Input: dimensioned drawing with shaded views. Units: mm. Origin: part minimum x, y, z. A direction names the side the tool comes from. Give positions to 0.01 mm unless a question says otherwise; leave off trailing zeros. Loops run counter-clockwise (first coordinate to the right, second up) from the corner with the lowest first, then second, coordinate; pieces in that order, holes last.
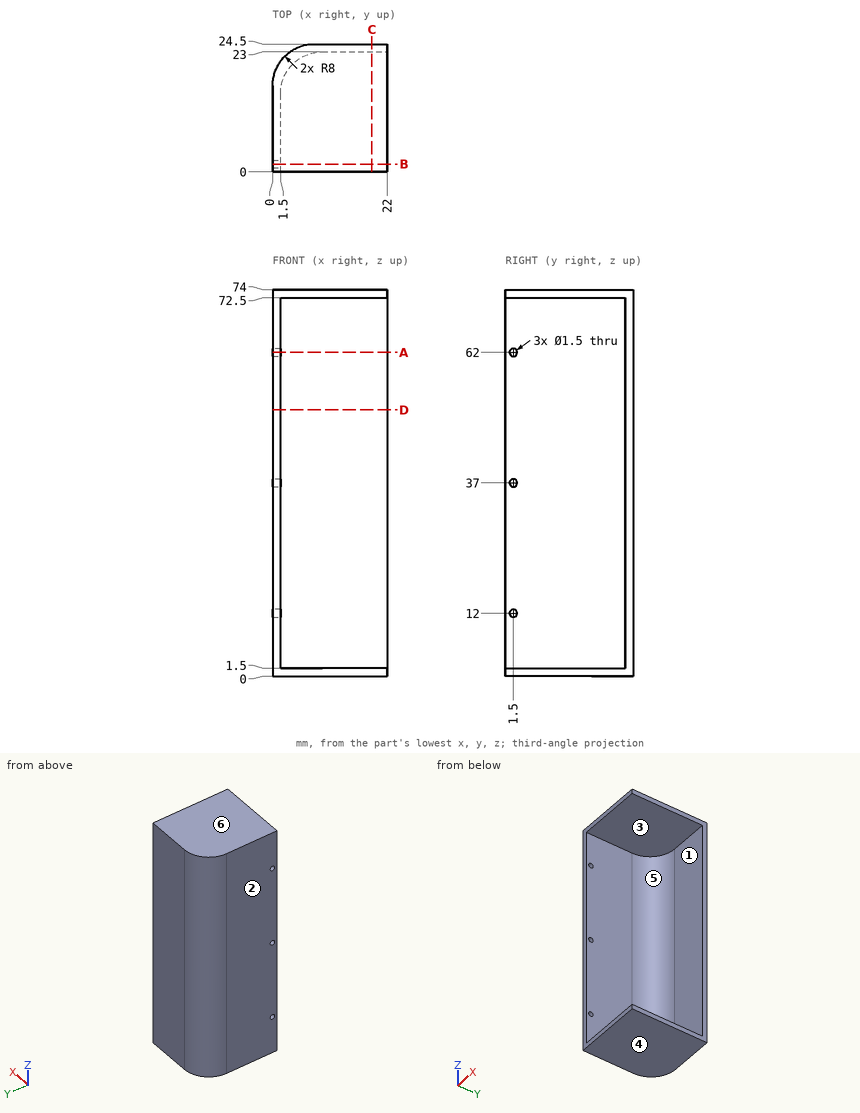
Item 1: Set-up query: the marked faces 5 and 6. Return all of +Z, -Z, +X, -X, +Y, -Y with unobstructed straight access to the full face (end or side cutting, diameter ignored); none if empty.
Values follow:
face 5: +X, -Y
face 6: +Z, +X, -X, +Y, -Y
Item 2: Section query A-A on z = 62. Return loops of the section in (x, y).
Values follow:
outline: (0, 0) - (1.5, 0) - (1.5, 0.75) - (0, 0.75) - close; (0, 2.25) - (1.5, 2.25) - (1.5, 15) arc R8 cw to (9.5, 23) - (22, 23) - (22, 24.5) - (8, 24.5) arc R8 ccw to (0, 16.5) - close
Item 3: Section query D-D on z = 51. Return loops of the section in (x, y), plus the area to 3 significant figures.
Values follow:
outline: (0, 0) - (1.5, 0) - (1.5, 15) arc R8 cw to (9.5, 23) - (22, 23) - (22, 24.5) - (8, 24.5) arc R8 ccw to (0, 16.5) - close
area: 67.5 mm2
Item 4: Section query B-B on y = 1.5. Return loops of the section in (x, z), plus the area to 3 significant figures.
Values follow:
outline: (0, 0) - (22, 0) - (22, 1.5) - (1.5, 1.5) - (1.5, 11.25) - (0, 11.25) - close; (0, 12.75) - (1.5, 12.75) - (1.5, 36.25) - (0, 36.25) - close; (0, 37.75) - (1.5, 37.75) - (1.5, 61.25) - (0, 61.25) - close; (0, 62.75) - (1.5, 62.75) - (1.5, 72.5) - (22, 72.5) - (22, 74) - (0, 74) - close
area: 166 mm2
Item 5: Ray query, probe 1 along Z at (x, y) = (0.6, 1.5); probe 2 along Z at (x, y) = (20.5, 19.5); probe 3 along Y at (x, z) = (9, 13). Return the intervals inside material, ascending.
Values follow:
probe 1: z = 0 to 11.25, 12.75 to 36.25, 37.75 to 61.25, 62.75 to 74
probe 2: z = 0 to 1.5, 72.5 to 74
probe 3: y = 22.98 to 24.5
Item 6: Pin query (flat end, axial travel): pin 1 (1.7 mm diameter, centred on y = 1.5, z = 37, fed in from +X); pin 2 (4 mm diameter, centred on x = 15, z = 44.5, fed in from -Y); pin 3 (2 mm diameter, centred on y = 21, z = 25.5, fed in from -X). Return the tip coordinate at first contact, or that it passes through.
Values follow:
pin 1: stops at x = 1.5
pin 2: stops at y = 23
pin 3: stops at x = 0.81
Item 7: Draft query along Z for the marked faces 1, 2, 3 and 4. Return one class per face: +Z half, -Z half, draft (parallel to the pull), parting line (faces both ways), or undercut.
Values follow:
face 1: undercut
face 2: draft
face 3: undercut
face 4: -Z half
Item 8: Section query C-C on x = 19. Return loops of the section in (y, z), plus the area to 3 significant figures.
Values follow:
outline: (0, 0) - (24.5, 0) - (24.5, 74) - (0, 74) - (0, 72.5) - (23, 72.5) - (23, 1.5) - (0, 1.5) - close
area: 180 mm2
